Check sheet for the modelled part. Datum: model origin and axes. Units: mm. Face numbers are marked on the shaded views. A direction names the side the tool comes from. Round coordinates to 2 decimals unless told otherwise and drop trailing zeros. Order: outer loops, then holes, each group sorted by start corner. A loop starts at its lowest first (then second) coordinate and runs counter-clockwise, first axis right, second up. Notation, with made-up numbers: (85.25, 45) -> (131.25, 45) arc R21 cw to (131.25, 78) -> close; hole circle Ø6 at (26, 81). An arc over 180 degrees is marked (long way). Answer in a Markdown table with one row per item. Add a question column.
1. Sectioned sample at B-B, the plane z = 19. Record the boundary of the cut face in (x, y).
2. Access from +Z, -Z, +X, -X, +Y, -Y to the whole of each face (thin tool, end or side, straight path). Record for the marked faces 1, 2 and 3.
3. Depth check by flat-ended pin: P1, Ø3, axis at x = -0.5, z = 8, coming from the -Y side; P2, Ø1.5, axis at x = 2, y = 3, coming from the +Z side; P3, Ø3, axis at x = 0, z = 19, coming from the +Y side. Enter the tip coordinate at first touch or a pass-through.
4. Sectioned sample at D-D, the plane y = 0.5. Record the boundary of the cut face in (x, z).
5. Sectioned sample at C-C, the plane z = 6.75. Record the boundary of the cut face in (x, y).
6. Sectioned sample at A-A, the plane x = 0. Record the boundary of the cut face in (y, z), then the cut area to 3 significant figures.
7. Material ranges on L1, parallel to Z at x = 0, y = 1.85; L2, parallel to Z at x = -1.5, y = -0.75; L3, parallel to Y at x = 1, z = 12.25, recorded low to high. Write a range as from..to.
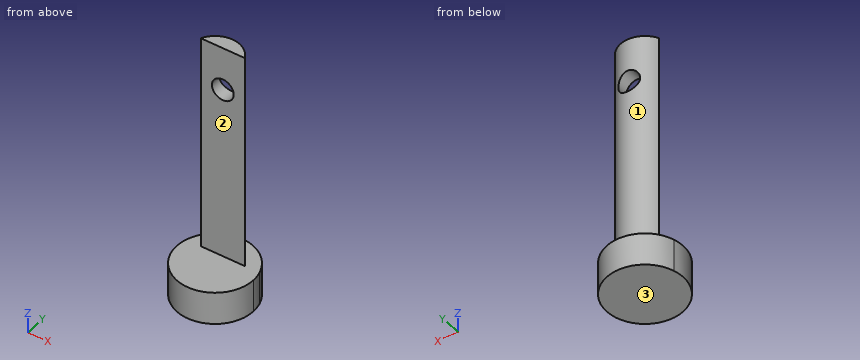
```python
from build123d import *

# Parameters (mm, degrees)
BOSS_EXTRUDE1_DEPTH = 3
BOSS_EXTRUDE2_DEPTH = 20
SKETCH3_R           = 1
CUT_EXTRUDE1_DEPTH  = 10


with BuildPart() as part:
    # Sketch1 → Boss-Extrude1 (new body)
    with BuildSketch(Plane.XY):
        with BuildLine():
            ThreePointArc((3.354101966, 1), (0, 3.5), (-3.354101966, 1))
            Line((-3.354101966, 1), (3.354101966, 1))
        make_face()
        with BuildLine():
            Line((3.354101966, 1), (-3.354101966, 1))
            ThreePointArc((-3.354101966, 1), (-0.505293538, -3.463333429), (3.5, 0))
            ThreePointArc((3.5, 0), (3.463333429, 0.505293538), (3.354101966, 1))
        make_face()
    extrude(amount=BOSS_EXTRUDE1_DEPTH)

    # Sketch2 → Boss-Extrude2 (add)
    with BuildSketch(Plane.XY.offset(3)):
        with BuildLine():
            ThreePointArc((2.015564437, 1), (0, 2.25), (-2.015564437, 1))
            Line((-2.015564437, 1), (2.015564437, 1))
        make_face()
    extrude(amount=BOSS_EXTRUDE2_DEPTH)

    # Sketch3 → Cut-Extrude1 (cut)
    with BuildSketch(Plane(origin=(0, 1, 0), x_dir=(-1, 0, 0), z_dir=(0, -1, 0))):
        with Locations(Location((0, -19, 0), (0, 0, 90))):
            Circle(SKETCH3_R)
    extrude(amount=-CUT_EXTRUDE1_DEPTH, mode=Mode.SUBTRACT)


solid = part.part
```
Answer key:
| question | item | result |
|---|---|---|
| 1 | outline | (-2.02, 1) -> (-1, 1) -> (-1, 2.02) arc R2.25 ccw to start; (1, 1) -> (2.02, 1) arc R2.25 ccw to (1, 2.02) -> close |
| 2 | face 1 | +Z, +Y |
| 2 | face 2 | +Z, +X, -X, -Y |
| 2 | face 3 | -Z, +X, -X, +Y, -Y |
| 3 | P1 | stops at y = 1 |
| 3 | P2 | stops at z = 3 |
| 3 | P3 | stops at y = 2.25 |
| 4 | outline | (-3.46, 0) -> (3.46, 0) -> (3.46, 3) -> (-3.46, 3) -> close |
| 5 | outline | (-2.02, 1) -> (2.02, 1) arc R2.25 ccw to start |
| 6 | outline | (-3.5, 0) -> (3.5, 0) -> (3.5, 3) -> (2.25, 3) -> (2.25, 18) -> (1, 18) -> (1, 3) -> (-3.5, 3) -> close; (1, 20) -> (2.25, 20) -> (2.25, 23) -> (1, 23) -> close |
| 6 | area | 43.5 mm² |
| 7 | L1 | z = 0..18, 20..23 |
| 7 | L2 | z = 0..3 |
| 7 | L3 | y = 1..2.02 |
